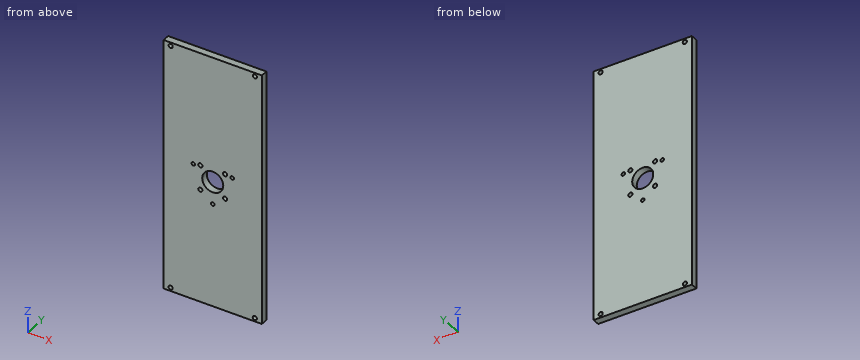
Autodesk Inventor part; units mm, degrees
ref_plane "YZ Plane" through (0, 0, 0) normal (1, 0, 0) x (0, 1, 0)
ref_plane "XZ Plane" through (0, 0, 0) normal (0, 1, 0) x (-1, 0, 0)
ref_plane "XY Plane" through (0, 0, 0) normal (0, 0, 1) x (1, 0, 0)
sketch "Sketch1" plane through (0, 0, 0) normal (0, 1, 0) x (-1, 0, 0)
  line L0 (35, 90) -> (-35, 90)
  line L1 (-35, 90) -> (-35, -90)
  line L2 (-35, -90) -> (35, -90)
  line L3 (35, -90) -> (35, 90)
  line L4 (69.6704, 0) -> (-52.4451, 0)
  line L5 (0, -129.3465) -> (0, 126.5577)
  point P0 (0, 0)
  dimension "d0" = 180
  dimension "d1" = 70
extrude "Extrusion1" add sketch "Sketch1" along normal blind 5
sketch "Sketch2" plane through (0, 5, 0) normal (0, 1, 0) x (1, 0, 0)
  line L0 (-35, 90) -> (-35, -90)
  line L1 (35, -90) -> (35, 90)
  line L2 (-35, -90) -> (35, -90)
  line L3 (-35, -90) -> (35, -90)
  line L4 (35, -90) -> (35, 90)
  line L5 (35, 90) -> (-35, 90)
  line L6 (-35, 90) -> (-35, -90)
  line L7 (-49, 0) -> (49, 0)
  line L8 (0, 126) -> (0, -126)
  point P0 (0, 0)
  point P1 (-30, -87.5)
  point P2 (-30, 87.5)
  point P3 (30, -87.5)
  point P4 (30, 87.5)
  dimension "d4" = 5
  dimension "d5" = 2.5
hole "Hole1" at (-30, 5, -87.5) at (30, 5, 87.5) at (30, 5, -87.5) at (-30, 5, 87.5) direction (0, -1, 0) diameter 3 depth 8.8 tip angle 118
sketch "Sketch3" plane through (0, 5, 0) normal (0, 1, 0) x (1, 0, 0)
  point P0 (0, 0)
hole "Hole2" at (0, 5, 0) direction (0, -1, 0) diameter 15 depth 14.2 tip angle 118
sketch "Sketch4" plane through (0, 5, 0) normal (0, 1, 0) x (1, 0, 0)
  circle A0 centre (0, 0) radius 7.5
  line L0 (35, 90) -> (-35, 90)
  line L1 (-35, 90) -> (-35, -90)
  line L2 (-35, -90) -> (35, -90)
  circle A1 centre (0, 0) radius 12.5
  line L3 (-35, 0) -> (35, 0)
  line L4 (35, -90) -> (35, 90)
  line L5 (0, 90) -> (0, -90)
  point P0 (-8.8388, -8.8388)
  point P1 (8.8388, -8.8388)
  point P2 (-8.8388, 8.8388)
  point P3 (8.8388, 8.8388)
  dimension "d42" = 25
  dimension "d45" = 45
hole "Hole3" at (-8.8388, 5, 8.8388) at (-8.8388, 5, -8.8388) at (8.8388, 5, -8.8388) at (8.8388, 5, 8.8388) direction (0, -1, 0) diameter 3 end through all
sketch "Sketch5" plane through (0, 5, 0) normal (0, 1, 0) x (1, 0, 0)
  point P0 (0, 0)
sketch "Sketch6" plane through (0, 5, 0) normal (0, 1, 0) x (1, 0, 0)
  point P0 (0, 0)
  point P1 (0, 16)
  point P2 (-13.8564, -8)
  point P3 (0, 0)
  point P4 (13.8564, -8)
  point P5 (0, 0)
  dimension "d30" = 16
  dimension "d33" = 360
hole "Hole4" at (-13.8564, 5, 8) at (13.8564, 5, 8) at (0, 5, -16) direction (0, -1, 0) diameter 2.5 end through all
properties part number "옆판" material "Aluminum 6061-AHC"
Can you work these out from the model? Positions are in its coordinate system, mm. Coordinates: 2 decimals unless noted, no trailing zeros. Write each loop counter-clockwise with the first axis right and the second up, starting at its lowest first coordinate (ties: lowest second). Pieces come first, ordered by that corner, then holes. Notation, with made-up numbers: (89.5, -13) -> (123.5, -13) arc R21 ccw to (123.5, -3) -> close; hole circle Ø11 at (57.25, 50.25). An arc over 180 degrees is marked (long way). Answer as CSV lines item,"result".
1) If we section it at B-B on y = 1.5: Count the separate pieces of the cut face and the enclosed holes in it, then the cut area to 3 significant figures.
Check result:
separate pieces,"1"
enclosed holes,"12"
area,"12,400 mm²"
2) If I drill on line 1 (Z direction, x = 30, y = 3.2); line 2 (Z direction, x = 0, y = 2.9); line 3 (X direction, y = 3.4, z = 0), over which ranges is the centre line in solid material (lowest first)? Write a range as from..to.
Check result:
line 1,"-90..-89, -86..86, 89..90"
line 2,"-90..-17.25, -14.75..-7.5, 7.5..90"
line 3,"-35..-7.5, 7.5..35"
3) If we section it at A-A on z = 0: Please give me the cut outline in (x, y), then the cut area to 3 significant figures.
Check result:
outline,"(-35, 0) -> (-7.5, 0) -> (-7.5, 5) -> (-35, 5) -> close; (7.5, 0) -> (35, 0) -> (35, 5) -> (7.5, 5) -> close"
area,"275 mm²"
